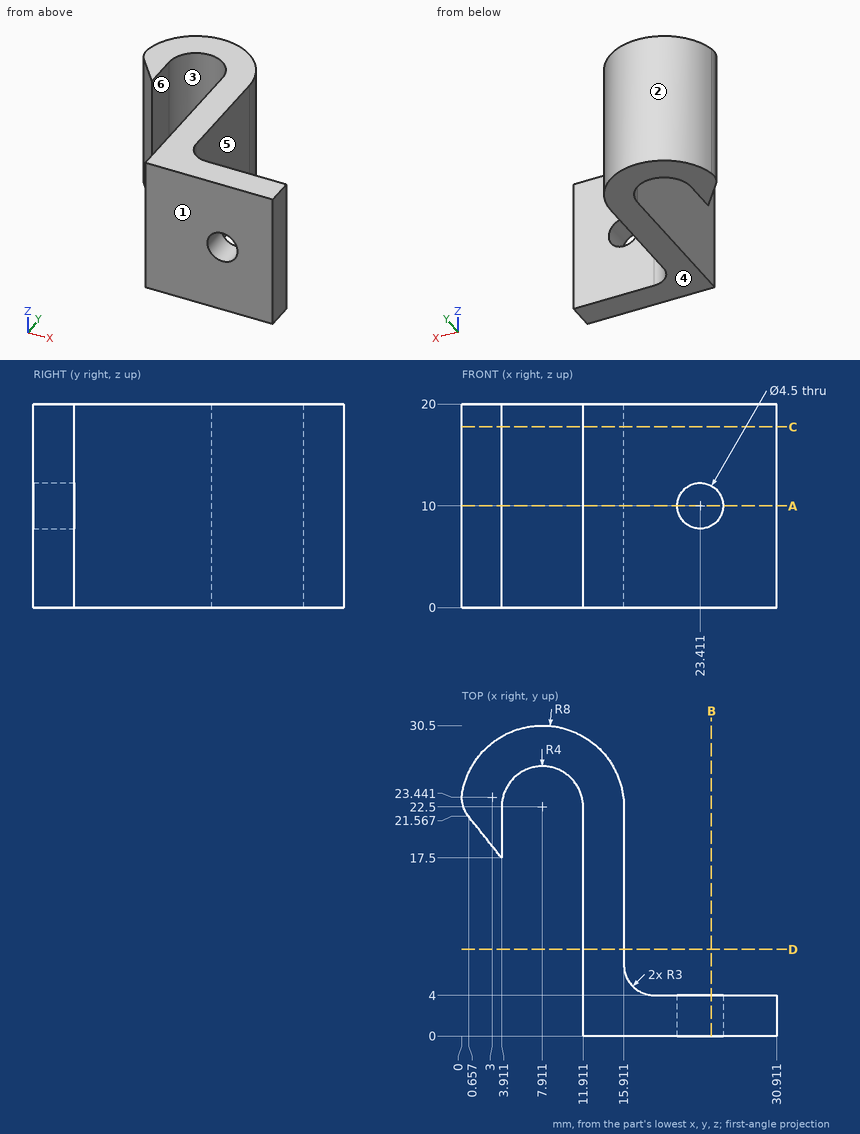
Verification items for this drawing (mm, ordinates from the low corner). A direction names the side the tool comes from. Coordinates: 2 decimals unless noted, no trailing zeros. Loops run counter-clockwise (first coordinate to the right, second up) from the corner with the lowest first, then second, coordinate; pieces in that order, holes last.
Item 1: Go/stop test with flat-tipped pins: pin 1 Ø9.5 at (x, z) = (23, 6) entering from +Y; pin 2 Ø3 at (y, z) = (6, 13) entering from -X; pin 3 Ø1.5 at (x, y) = (12.5, 19) entering from -Z; pin 4 Ø4.5 at (y, z) = (18.5, 8.5) entering from +X. Record where each tip stops, or that it passes through.
Item 2: Thickness scan on line 1 (X direction, y = 3, z = 10); line 2 (Y direction, x = 21.5, z = 15.75); line 3 (X direction, y = 16, z = 16.75). Record the ranges inside material, lowest first.
Item 3: Sectioned sample at A-A, the plane z = 10. Record the boundary of the cut face in (x, y) (1 decimal), then the cut area to 3 significant figures.
Item 4: Sectioned sample at D-D, the plane y = 8.5. Record the boundary of the cut face in (x, z), then the cut area to 3 significant figures.
Item 5: Sectioned sample at B-B, the plane x = 24.5. Record the boundary of the cut face in (y, z).
Item 6: Sectioned sample at C-C, the plane z = 17.75. Record the boundary of the cut face in (x, y) (1 decimal), then the cut area to 3 significant figures.
Item 7: Release check for a two-part mould opening along X. For the marked faces 1, 2 and 3 record: released by +X, released by -X, zero draft, split by the parting line, or undercut.
Item 8: Access from +Z, -Z, +X, -X, +Y, -Y to the whole of each face (thin tool, end or side, straight path). Record for the marked faces 4, 5 and 6.
Check result:
1. pin 1: stops at y = 4.07
1. pin 2: stops at x = 11.91
1. pin 3: stops at z = 0
1. pin 4: stops at x = 15.91
2. line 1: x = 11.91 to 21.16, 25.66 to 30.91
2. line 2: y = 0 to 4
2. line 3: x = 11.91 to 15.91
3. outline: (0.1, 24) arc R3 ccw to (0.7, 21.6) - (3.9, 17.5) - (3.9, 22.5) arc R4 cw to (11.9, 22.5) - (11.9, 0) - (21.2, 0) - (21.2, 4) - (18.9, 4) arc R3 cw to (15.9, 7) - (15.9, 22.5) arc R8 ccw to start; (25.7, 0) - (30.9, 0) - (30.9, 4) - (25.7, 4) - close
3. area: 219 mm2
4. outline: (11.91, 0) - (15.91, 0) - (15.91, 20) - (11.91, 20) - close
4. area: 80.0 mm2
5. outline: (0, 0) - (4, 0) - (4, 8.03) - (0, 8.03) - close; (0, 11.97) - (4, 11.97) - (4, 20) - (0, 20) - close
6. outline: (0.1, 24) arc R3 ccw to (0.7, 21.6) - (3.9, 17.5) - (3.9, 22.5) arc R4 cw to (11.9, 22.5) - (11.9, 0) - (30.9, 0) - (30.9, 4) - (18.9, 4) arc R3 cw to (15.9, 7) - (15.9, 22.5) arc R8 ccw to start
6. area: 237 mm2
7. face 1: zero draft
7. face 2: split by the parting line
7. face 3: undercut
8. face 4: -Z, +X, -X, +Y, -Y
8. face 5: +Z, -Z, +X, +Y
8. face 6: +Z, -Z, -Y
